from build123d import *

# Parameters (mm, degrees)
SKETCH_1_W          = 51
SKETCH_1_H          = 153
EXTRUDE_1_DEPTH     = 1
SKETCH_2_R          = 1.6
CUT_EXTRUDE_1_DEPTH = 2
CHAMFER_1_SIZE      = 5
EXTRUDE_2_DEPTH     = 1


with BuildPart() as part:
    # 草图1 → 凸台-拉伸1 (new body)
    with BuildSketch(Plane(origin=(0, 0, 0), x_dir=(1, 0, 0), z_dir=(0, 1, 0))):
        Rectangle(SKETCH_1_W, SKETCH_1_H)
    extrude(amount=EXTRUDE_1_DEPTH)

    # 草图2 → 切除-拉伸1 (cut, through all)
    with BuildSketch(Plane(origin=(0, 1, 0), x_dir=(1, 0, 0), z_dir=(0, 1, 0))):
        with Locations((-7, -70.5)):
            Circle(SKETCH_2_R)
        with Locations((7, -70.5)):
            Circle(SKETCH_2_R)
        with BuildLine():
            Line((-10, 63.5), (-10, -56.5))
            ThreePointArc((-10, -56.5), (-14, -60.5), (-18, -56.5))
            Line((-18, -56.5), (-18, 63.5))
            ThreePointArc((-18, 63.5), (-14, 67.5), (-10, 63.5))
        make_face()
        with BuildLine():
            Line((4, 63.5), (4, -56.5))
            ThreePointArc((4, -56.5), (0, -60.5), (-4, -56.5))
            Line((-4, -56.5), (-4, 63.5))
            ThreePointArc((-4, 63.5), (0, 67.5), (4, 63.5))
        make_face()
        with BuildLine():
            Line((18, 63.5), (18, -56.5))
            ThreePointArc((18, -56.5), (14, -60.5), (10, -56.5))
            Line((10, -56.5), (10, 63.5))
            ThreePointArc((10, 63.5), (14, 67.5), (18, 63.5))
        make_face()
    extrude(amount=-CUT_EXTRUDE_1_DEPTH, mode=Mode.SUBTRACT)

    # 倒角1
    chamfer_1_edges = [part.edges().sort_by_distance(p)[0] for p in [
        (-25.5, 0.5, -76.5),
        (25.5, 0.5, -76.5),
        (25.5, 0.5, 76.5),
        (-25.5, 0.5, 76.5),
    ]]
    chamfer(chamfer_1_edges, length=CHAMFER_1_SIZE)

    # 草图4 → 凸台-拉伸2 (add)
    with BuildSketch(Plane(origin=(0, 1, 0), x_dir=(1, 0, 0), z_dir=(0, 1, 0))):
        with BuildLine():
            Line((-10, -56.5), (-10, 63.5))
            ThreePointArc((-10, 63.5), (-14, 67.5), (-18, 63.5))
            Line((-18, 63.5), (-18, -56.5))
            ThreePointArc((-18, -56.5), (-14, -60.5), (-10, -56.5))
        make_face()
        with BuildLine():
            Line((-11.6, 63.5), (-11.6, -56.5))
            ThreePointArc((-11.6, -56.5), (-14, -58.9), (-16.4, -56.5))
            Line((-16.4, -56.5), (-16.4, 63.5))
            ThreePointArc((-16.4, 63.5), (-14, 65.9), (-11.6, 63.5))
        make_face(mode=Mode.SUBTRACT)
    extrude(amount=-EXTRUDE_2_DEPTH)


solid = part.part
Design review of the part built by this model. Coordinates are the model's own, in mm. A direction names the side the tool comes from. Round coordinates to 2 decimals unless told otherwise and drop trailing zeros. Write each loop counter-clockwise with the first axis right and the second up, starting at its lowest first coordinate (ties: lowest second). Pieces come first, ordered by that corner, then holes. Notation, with made-up numbers: (-16.75, 49.5) - (20.25, 49.5) arc R15 cw to (20.25, 63.5) - close; hole circle Ø7 at (-36, -4). An arc over 180 degrees is marked (long way). Return JSON: item names as keys, results as strings. Group by question number.
Item 1: We need section C-C on y = 0.25. Write out the cut boundary in (x, z).
Item 2: Insertion check: P1, Ø5, axis at x = 3, z = 21.5, coming from the -Y side. The pin has a flat end and moves straight along its axis. Give the tip position at first contact, or say it passes through.
Item 3: We need section D-D on x = 16. Write out the cut boundary in (y, z), and give its area (3 significant figures).
Item 4: The part is to be moulded in two halves that separate along X. For faces 3 (the face through (23, 0.5, -74)), 4 (the face through (0.1, 0.5, 60.5)), 5 (the face through (-6, 1, -1)), say which applies: pulls with the +X half, pulls with the -X half, needs draft (parallel to the pull), parting line crosses it, or undercut.
Item 5: Machinability: for faces 1 (the face through (-23, 0.5, -74)), 2 (the face through (14.1, 0.5, 60.5)), which of the approach directions +Z, -Z, +X, -X, +Y, -Y give a long, thin tool a straight path to every point of the face, cutting with its end or side? Answer none if there is none.
Item 6: We need section B-B on z = 52. Write out the cut boundary in (x, y).
Item 7: For probe 1 along X at (y, z) = (0.55, 70.5); probe 2 along X at (y, z) = (0.5, 1.5); probe 3 along Z at (x, y) = (7, 0.5), list the stretches that pass through material, from the lowest coordinate up. Write a range as [from, to].
Item 8: We need section A-A on x = -14. Write out the cut boundary in (y, z).
Model answer:
{
 "1": {"outline": "(-25.5, -71.5) - (-20.5, -76.5) - (20.5, -76.5) - (25.5, -71.5) - (25.5, 71.5) - (20.5, 76.5) - (-20.5, 76.5) - (-25.5, 71.5) - close; hole (-16.4, -63.5) arc R2.4 ccw to (-11.6, -63.5) - (-11.6, 56.5) arc R2.4 ccw to (-16.4, 56.5) - close; hole circle Ø3.2 at (-7, 70.5); hole (-4, -63.5) arc R4 ccw to (4, -63.5) - (4, 56.5) arc R4 ccw to (-4, 56.5) - close; hole circle Ø3.2 at (7, 70.5); hole (10, -63.5) arc R4 ccw to (18, -63.5) - (18, 56.5) arc R4 ccw to (10, 56.5) - close"},
 "2": {"P1": "stops at y = 0"},
 "3": {"outline": "(0, -76.5) - (1, -76.5) - (1, -66.96) - (0, -66.96) - close; (0, 59.96) - (1, 59.96) - (1, 76.5) - (0, 76.5) - close", "area": "26.1 mm²"},
 "4": {"face 3": "pulls with the +X half", "face 4": "undercut", "face 5": "needs draft"},
 "5": {"face 1": "-Z, -X, +Y, -Y", "face 2": "+Y, -Y"},
 "6": {"outline": "(-25.5, 0) - (-16.4, 0) - (-16.4, 1) - (-25.5, 1) - close; (-11.6, 0) - (-4, 0) - (-4, 1) - (-11.6, 1) - close; (4, 0) - (10, 0) - (10, 1) - (4, 1) - close; (18, 0) - (25.5, 0) - (25.5, 1) - (18, 1) - close"},
 "7": {"probe 1": "x = [-25.5, -8.6], [-5.4, 5.4], [8.6, 25.5]", "probe 2": "x = [-25.5, -16.4], [-11.6, -4], [4, 10], [18, 25.5]", "probe 3": "z = [-76.5, 68.9], [72.1, 76.5]"},
 "8": {"outline": "(0, -76.5) - (1, -76.5) - (1, -65.9) - (0, -65.9) - close; (0, 58.9) - (1, 58.9) - (1, 76.5) - (0, 76.5) - close"}
}
